Geometry: final body of the model. Coordinates: model frame, mm. A direction names the side the tool comes from. Round coordinates to 2 decimals unless told otherwise and drop trailing zeros. Loops run counter-clockwise (first coordinate to the right, second up) from the corner with the lowest first, then second, coordinate; pieces in that order, holes last. Notation, with made-up numbers: (61, 15) - (80, 15) arc R25 ccw to (80, 54) - close; hole circle Ø11 at (40, -33). An arc over 180 degrees is marked (long way). Return JSON: item names as keys, results as strings. Group by question number.
1. Section C-C on z = 1.15. Return loops of the section in (x, y).
2. Section B-B on y = 73.75. Return loops of the section in (x, z).
3. Set-up query: faces 1 (the face through (15.805, 87.057, 2.958)), 2 (the face through (22.089, 74.604, 3.972)). Return all of +Z, -Z, +X, -X, +Y, -Y with unobstructed straight access to the full face (end or side cutting, diameter ignored); none if empty.
4. First-contact query: pin 1 Ø1 at (y, z) = (79, 4) entering from +X; pin 2 Ø6 at (x, y) = (23.5, 82) entering from +Z. Flat tips, straight axial feed; report the tip coordinate or a pass-through.
5. Section D-D on y = 84.25. Return loops of the section in (x, z), and give its area (3 significant figures).
6. Draft query along Y for faces 3 (the face through (24.5, 78.5, 2)), 4 (the face through (21.37, 69.15, 2.96)), 5 (the face through (28, 76, 6)). Return one class per face: +Y half, -Y half, draft (parallel to the pull), parting line (faces both ways), or undercut.
7. Section A-A on x = 23. Return loops of the section in (y, z).
8. Material intervals for probe 1 along X at (y, z) = (73.5, 4.55); probe 2 along X at (y, z) = (75.5, 3.7); probe 3 along Y at (x, z) = (30.25, 0.4), sorted ascending.
Autodesk Inventor part; units mm, degrees
ref_plane "YZ Plane" through (0, 0, 0) normal (1, 0, 0) x (0, 1, 0)
ref_plane "XZ Plane" through (0, 0, 0) normal (0, 1, 0) x (-1, 0, 0)
ref_plane "XY Plane" through (0, 0, 0) normal (0, 0, 1) x (1, 0, 0)
ref_plane "РабПлоскость1" through (0, 0, 0) normal (0, 0, 1) x (1, 0, 0)
sketch "Эскиз1" plane through (0, 0, 0) normal (0, 0, 1) x (1, 0, 0)
  circle A0 centre (30, 88.544) radius 1.5
  circle A1 centre (30, 74.544) radius 1.5
  circle A2 centre (16, 74.544) radius 1.5
  circle A3 centre (16, 88.544) radius 1.5
  circle A4 centre (23, 81.544) radius 7
  circle A5 centre (23, 81.544) radius 12.5
  circle A6 centre (23, 81.544) radius 3
  point P0 (0, 0)
  dimension "d0" = 25
  dimension "d5" = 6
extrude "Выдавливание1" add sketch "Эскиз1" along normal blind 6 contours A5
extrude "Выдавливание2" add sketch "Эскиз1" along normal blind 2 contours A4
properties part number "подшипник не выпадет"
Taken from the geometry:
{
 "1": {"outline": "circle Ø25 at (23, 81.54); hole circle Ø3 at (16, 74.54); hole circle Ø3 at (16, 88.54); hole circle Ø6 at (23, 81.54); hole circle Ø3 at (30, 74.54); hole circle Ø3 at (30, 88.54)"},
 "2": {"outline": "(13.23, 0) - (14.73, 0) - (14.73, 6) - (13.23, 6) - close; (17.27, 0) - (28.73, 0) - (28.73, 6) - (17.27, 6) - close; (31.27, 0) - (32.77, 0) - (32.77, 6) - (31.27, 6) - close"},
 "3": {"face 1": "+Z, -Z", "face 2": "+Z"},
 "4": {"pin 1": "x = 35.33", "pin 2": "z = 2"},
 "5": {"outline": "(10.8, 0) - (21.7, 0) - (21.7, 2) - (16.54, 2) - (16.54, 6) - (10.8, 6) - close; (24.3, 0) - (35.2, 0) - (35.2, 6) - (29.46, 6) - (29.46, 2) - (24.3, 2) - close", "area": "89.6 mm2"},
 "6": {"face 3": "undercut", "face 4": "parting line", "face 5": "draft"},
 "7": {"outline": "(69.04, 0) - (78.54, 0) - (78.54, 2) - (74.54, 2) - (74.54, 6) - (69.04, 6) - close; (84.54, 0) - (94.04, 0) - (94.04, 6) - (88.54, 6) - (88.54, 2) - (84.54, 2) - close"},
 "8": {"probe 1": "13.43 to 14.92, 17.08 to 28.92, 31.08 to 32.57", "probe 2": "12.06 to 14.84, 17.16 to 19.47, 26.53 to 28.84, 31.16 to 33.94", "probe 3": "71.36 to 73.06, 76.02 to 87.06, 90.02 to 91.73"}
}
